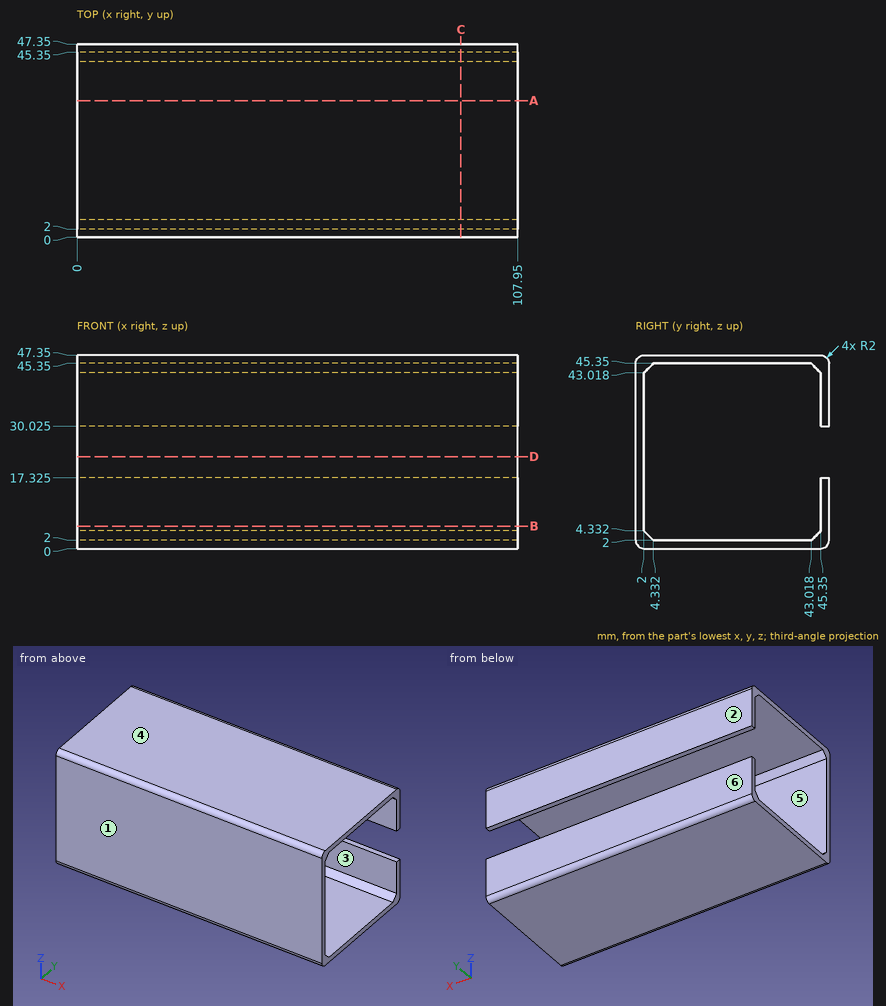
Source: three-view drawing plus pictorial views. Frame: mm from the lowest corner of the part. A direction names the side the tool comes from. Give positions to 0.01 mm unless a question says otherwise; leave off trailing zeros. Loops run counter-clockwise (first coordinate to the right, second up) from the corner with the lowest first, then second, coordinate; pieces in that order, holes last.
1) Line query: L1, parallel to Z at x = 56.5, y = 9; L2, parallel to Z at x = 49, y = 45.5 (1 decimal). Output: solid intervals per line, ascending.
A:
L1: z = 0 to 2, 45.35 to 47.35
L2: z = 0 to 17.3, 30 to 47.3
2) Section query C-C on x = 94. Return the cut outline in (y, z) (3 decimals), and give its area (3 significant figures).
A:
outline: (0, 2) arc R2 ccw to (2, 0) - (45.35, 0) arc R2 ccw to (47.35, 2) - (47.35, 17.325) - (45.35, 17.325) - (45.35, 4.332) - (43.018, 2) - (4.332, 2) - (2, 4.332) - (2, 43.018) - (4.332, 45.35) - (43.018, 45.35) - (45.35, 43.018) - (45.35, 30.025) - (47.35, 30.025) - (47.35, 45.35) arc R2 ccw to (45.35, 47.35) - (2, 47.35) arc R2 ccw to (0, 45.35) - close
area: 345 mm2
3) Mould query, pull axis Y, two halves, no side actions, for the marked faces 1, 2, 3 and 4. Classes: released by +Y, released by -Y, zero draft, split by the parting line, or undercut.
A:
face 1: released by -Y
face 2: released by +Y
face 3: undercut
face 4: zero draft
4) Contact query for flat-ended pins moving along their axis: pin 1 (12 mm diameter, centred on y = 9, z = 23, fed in from -X); pin 2 (2 mm diameter, centred on x = 74, y = 46.5, fed in from +Z); pin 3 (1 mm diameter, centred on x = 54, y = 46, fed in from -Z). Output: stop coordinate, or through.
A:
pin 1: passes through
pin 2: stops at z = 47.34
pin 3: stops at z = 0.01
5) Reachability of the marked faces 5 and 6 from +Z, -Z, +X, -X, +Y, -Y: full face, straight path, thin tool, end or side. Return the list, or none.
A:
face 5: +X, -X
face 6: +Z, -Z, +X, -X, +Y
6) Section query A-A on y = 33.5. Return the cut outline in (x, z).
A:
outline: (0, 0) - (107.95, 0) - (107.95, 2) - (0, 2) - close; (0, 45.35) - (107.95, 45.35) - (107.95, 47.35) - (0, 47.35) - close
7) Section query D-D on z = 22.5. Return the cut outline in (x, y), and give its area (3 significant figures).
A:
outline: (0, 0) - (107.95, 0) - (107.95, 2) - (0, 2) - close
area: 216 mm2
